The model under review builds one solid part; all positions refer to its coordinate system, in mm. A direction names the side the tool comes from. Round coordinates to 2 decimals unless told otherwise and drop trailing zeros. Write each loop counter-clockwise with the first axis right and the second up, starting at its lowest first coordinate (ties: lowest second). Pieces come first, ordered by that corner, then holes. Notation, with made-up numbers: (-35, 22.25) -> (-14, 22.25) arc R25 cw to (-14, 40.25) -> close; hole circle Ø2 at (76.25, -10.5). An arc over 180 degrees is marked (long way). Answer as a JSON object with one key per item and string values. Group by question number.
1) We need section B-B, the plane z = 0. Write out the cut boundary in (x, y), then the cut area to 4 significant figures.
2) We need section C-C, the plane x = -39. Write out the cut boundary in (y, z).
3) Insertion check: pin 1 Ø1 at (x, y) = (-22.5, 19) entering from -Z; pin 2 Ø3 at (x, y) = (17.5, 26.5) entering from +Z; pin 3 Ø10 at (y, z) = (67, -7) entering from +X. Each pin has a flat end and moves straight along its axis. Give the tip position at first contact, or say it passes through.
4) We need section D-D, the plane y = 26. Write out the cut boundary in (x, z), then the cut area to 3 significant figures.
5) Mouldability with a two-part tool opening along Z and no side actions: class faces 1 (the flat face through (-1, 15, -34)), 2 (the cylindrical face through (-0.862, 72.395, 35.995)), 3 (the cylindrical face through (-47.857, 72.395, -1.301)), 4 (the cylindrical face through (60, 72, 0)) as pulls with the +Z half, pulls with the -Z half, needs draft (parallel to the pull), parting line crosses it, or undercut.
6) To check wall thickness, follow probe 1 along X at (y, z) = (72.75, 0); probe 2 along X at (y, z) = (6, 0); probe 3 along Y at (x, z) = (25.5, -27.5). State the ranges of each line that lie inside material, in increasing order. Write a range as [from, to].
7) We need section A-A, the plane x = 0. Write out the cut boundary in (y, z).
8) Machinability: for faces 5 (the cylindrical face through (-32.215, 39.65, -7.154)), 6 (the cylindrical face through (-60, 72, 0)), 7 (the cylindrical face through (6.31, 47.96, 20.03)), which of the approach directions +Z, -Z, +X, -X, +Y, -Y give a long, thin tool a straight path to every point of the face, cutting with its end or side? Answer none if there is none.
from build123d import *

# Parameters (mm, degrees)
SKETCH1_W           = 160
SKETCH1_H           = 100
BOSS_EXTRUDE1_DEPTH = 15
SKETCH3_R           = 16.5
CUT_EXTRUDE1_DEPTH  = 15
SKETCH2_R           = 33
BOSS_EXTRUDE2_DEPTH = 50
SKETCH6_R           = 6
BOSS_EXTRUDE4_DEPTH = 15
SKETCH7_R           = 21
CUT_EXTRUDE3_DEPTH  = 65


with BuildPart() as part:
    # Sketch1 → Boss-Extrude1 (new body)
    with BuildSketch(Plane(origin=(0, 0, 0), x_dir=(1, 0, 0), z_dir=(0, 1, 0))):
        Rectangle(SKETCH1_W, SKETCH1_H)
    extrude(amount=BOSS_EXTRUDE1_DEPTH)

    # Sketch3 → Cut-Extrude1 (cut)
    with BuildSketch(Plane.XZ):
        with Locations(Location((0, 0, 0), (0, 0, 270))):
            Circle(SKETCH3_R)
    extrude(amount=-CUT_EXTRUDE1_DEPTH, mode=Mode.SUBTRACT)

    # Sketch2 → Boss-Extrude2 (add)
    with BuildSketch(Plane(origin=(0, 15, 0), x_dir=(1, 0, 0), z_dir=(0, 1, 0))):
        with Locations(Location((0, 0, 0), (0, 0, 270))):
            Circle(SKETCH2_R)
    extrude(amount=BOSS_EXTRUDE2_DEPTH)

    # Sketch6 → Boss-Extrude4 (add)
    with BuildSketch(Plane(origin=(0, 65, 0), x_dir=(1, 0, 0), z_dir=(0, 1, 0))):
        with BuildLine():
            ThreePointArc((-55.034482759, 12.413793103), (-60, 0), (-55.034482759, -12.413793103))
            ThreePointArc((-55.034482759, -12.413793103), (0, -36), (55.034482759, -12.413793103))
            ThreePointArc((55.034482759, -12.413793103), (60, 0), (55.034482759, 12.413793103))
            ThreePointArc((55.034482759, 12.413793103), (0, 36), (-55.034482759, 12.413793103))
        make_face()
        with Locations(Location((-42, 0, 0), (0, 0, 270))):
            Circle(SKETCH6_R, mode=Mode.SUBTRACT)
        with Locations(Location((42, 0, 0), (0, 0, 270))):
            Circle(SKETCH6_R, mode=Mode.SUBTRACT)
    extrude(amount=BOSS_EXTRUDE4_DEPTH)

    # Sketch7 → Cut-Extrude3 (cut)
    with BuildSketch(Plane(origin=(0, 80, 0), x_dir=(1, 0, 0), z_dir=(0, 1, 0))):
        with Locations(Location((0, 0, 0), (0, 0, 270))):
            Circle(SKETCH7_R)
    extrude(amount=-CUT_EXTRUDE3_DEPTH, mode=Mode.SUBTRACT)


solid = part.part
Here are the results:
{
 "1": {"outline": "(-80, 0) -> (-16.5, 0) -> (-16.5, 15) -> (-21, 15) -> (-21, 80) -> (-36, 80) -> (-36, 65) -> (-33, 65) -> (-33, 15) -> (-80, 15) -> close; (-60, 65) -> (-48, 65) -> (-48, 80) -> (-60, 80) -> close; (16.5, 0) -> (80, 0) -> (80, 15) -> (33, 15) -> (33, 65) -> (36, 65) -> (36, 80) -> (21, 80) -> (21, 15) -> (16.5, 15) -> close; (48, 65) -> (60, 65) -> (60, 80) -> (48, 80) -> close", "area": "3,915 mm^2"},
 "2": {"outline": "(0, -50) -> (15, -50) -> (15, 50) -> (0, 50) -> close; (65, -25.23) -> (80, -25.23) -> (80, -5.2) -> (65, -5.2) -> close; (65, 5.2) -> (80, 5.2) -> (80, 25.23) -> (65, 25.23) -> close"},
 "3": {"pin 1": "stops at z = -24.6", "pin 2": "stops at z = 28.86", "pin 3": "stops at x = 59.89"},
 "4": {"outline": "circle Ø66 at (0, 0); hole circle Ø42 at (0, 0)", "area": "2,040 mm^2"},
 "5": {"face 1": "needs draft", "face 2": "pulls with the +Z half", "face 3": "undercut", "face 4": "parting line crosses it"},
 "6": {"probe 1": "x = [-60, -48], [-36, -21], [21, 36], [48, 60]", "probe 2": "x = [-80, -16.5], [16.5, 80]", "probe 3": "y = [0, 15], [65, 80]"},
 "7": {"outline": "(0, -50) -> (15, -50) -> (15, -33) -> (65, -33) -> (65, -36) -> (80, -36) -> (80, -21) -> (15, -21) -> (15, -16.5) -> (0, -16.5) -> close; (0, 16.5) -> (15, 16.5) -> (15, 21) -> (80, 21) -> (80, 36) -> (65, 36) -> (65, 33) -> (15, 33) -> (15, 50) -> (0, 50) -> close"},
 "8": {"face 5": "none", "face 6": "-X, +Y", "face 7": "+Y"}
}
